Read the model definition and answer for the solid it produces. Units are mm, in the model's axes. Face numbers are marked on the shaded views. A direction names the side the tool comes from. Round coordinates to 2 decimals unless told otherwise and drop trailing zeros. Loops run counter-clockwise (first coordinate to the right, second up) from the corner with the lowest first, then second, coordinate; pieces in that order, holes last. Notation, with made-up numbers: M -31,-3.75 L 10,-3.75 A8 cw 10,1.25 Z; hole C 3,28 d3. An arc over 180 degrees is marked long. Answer as CSV lines item,"result".
```python
from build123d import *

# Parameters (mm, degrees)
CROQUIS1_R              = 4.05
SALIENTE_EXTRUIR1_DEPTH = 15
CORTAR_EXTRUIR1_REACH   = 10
CROQUIS2_R              = 2.5
REDONDEO1_R             = 0.5
REDONDEO2_R             = 0.1


with BuildPart() as part:
    # Croquis1 → Saliente-Extruir1 (new body, symmetric)
    with BuildSketch(Plane.XY):
        with BuildLine():
            Line((21, 0), (-21, 0))
            Line((-21, 0), (-21, 8))
            Line((-21, 8), (-12, 8))
            Line((-12, 8), (-12, 20))
            ThreePointArc((-12, 20), (0, 32), (12, 20))
            Line((12, 20), (12, 8))
            Line((12, 8), (21, 8))
            Line((21, 8), (21, 0))
        make_face()
        with Locations((0, 20)):
            Circle(CROQUIS1_R, mode=Mode.SUBTRACT)
    extrude(amount=SALIENTE_EXTRUIR1_DEPTH, both=True)

    # Croquis2 → Cortar-Extruir1 (cut, up to next)
    with BuildSketch(Plane(origin=(0, 8, 0), x_dir=(1, 0, 0), z_dir=(0, 1, 0)), mode=Mode.PRIVATE) as cortar_extruir1_sk1:
        with Locations((-17.5, 11.25)):
            Circle(CROQUIS2_R)
    cortar_extruir1_tool1 = extrude(cortar_extruir1_sk1.sketch, amount=-CORTAR_EXTRUIR1_REACH, mode=Mode.PRIVATE) & part.part
    add(cortar_extruir1_tool1.solids().sort_by_distance((-17.5, 8, -11.25))[0], mode=Mode.SUBTRACT)
    # Croquis2 → Cortar-Extruir1 (cut, up to next)
    with BuildSketch(Plane(origin=(0, 8, 0), x_dir=(1, 0, 0), z_dir=(0, 1, 0)), mode=Mode.PRIVATE) as cortar_extruir1_sk2:
        with Locations((17.5, 11.25)):
            Circle(CROQUIS2_R)
    cortar_extruir1_tool2 = extrude(cortar_extruir1_sk2.sketch, amount=-CORTAR_EXTRUIR1_REACH, mode=Mode.PRIVATE) & part.part
    add(cortar_extruir1_tool2.solids().sort_by_distance((17.5, 8, -11.25))[0], mode=Mode.SUBTRACT)
    # Croquis2 → Cortar-Extruir1 (cut, up to next)
    with BuildSketch(Plane(origin=(0, 8, 0), x_dir=(1, 0, 0), z_dir=(0, 1, 0)), mode=Mode.PRIVATE) as cortar_extruir1_sk3:
        with Locations((-17.5, -11.25)):
            Circle(CROQUIS2_R)
    cortar_extruir1_tool3 = extrude(cortar_extruir1_sk3.sketch, amount=-CORTAR_EXTRUIR1_REACH, mode=Mode.PRIVATE) & part.part
    add(cortar_extruir1_tool3.solids().sort_by_distance((-17.5, 8, 11.25))[0], mode=Mode.SUBTRACT)
    # Croquis2 → Cortar-Extruir1 (cut, up to next)
    with BuildSketch(Plane(origin=(0, 8, 0), x_dir=(1, 0, 0), z_dir=(0, 1, 0)), mode=Mode.PRIVATE) as cortar_extruir1_sk4:
        with Locations((17.5, -11.25)):
            Circle(CROQUIS2_R)
    cortar_extruir1_tool4 = extrude(cortar_extruir1_sk4.sketch, amount=-CORTAR_EXTRUIR1_REACH, mode=Mode.PRIVATE) & part.part
    add(cortar_extruir1_tool4.solids().sort_by_distance((17.5, 8, 11.25))[0], mode=Mode.SUBTRACT)

    # Redondeo1
    redondeo1_edges = [part.edges().sort_by_distance(p)[0] for p in [
        (12, 14, -15),
        (16.5, 8, 15),
        (21, 4, 15),
        (-21, 4, 15),
        (-16.5, 8, 15),
        (-12, 14, 15),
        (0, 32, 15),
        (12, 14, 15),
        (0, 32, -15),
        (12, 8, 0),
        (21, 8, 0),
        (-21, 8, 0),
        (-12, 8, 0),
        (-12, 14, -15),
        (-16.5, 8, -15),
        (-21, 4, -15),
        (21, 4, -15),
        (16.5, 8, -15),
    ]]
    fillet(redondeo1_edges, radius=REDONDEO1_R)

    # Redondeo2
    redondeo2_edges = [part.edges().sort_by_distance(p)[0] for p in [
        (-4.05, 20, 15),
        (-4.05, 20, -15),
    ]]
    fillet(redondeo2_edges, radius=REDONDEO2_R)


solid = part.part
```
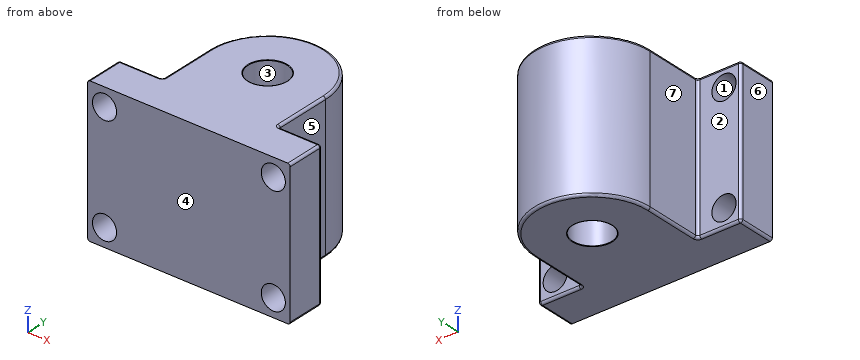
1) A tool of negligible diameter and unlimited length cuts with its end or side. For the marked faces 5, 6 and 7, from which of +Z, -Z, +X, -X, +Y, -Y can it reach the whole face along a straight path? Write none if from no direction.
Evaluation:
face 5,"+Z, -Z, +X, +Y"
face 6,"+Z, -Z, -X, +Y, -Y"
face 7,"+Z, -Z, -X, +Y"
2) Each of these flat-tipped pins is pushed along its axis until it touches: P1, Ø2, axis at x = 8, z = -0.5, coming from the +Y side; P2, Ø6.5, axis at x = -16, z = 7, coming from the +Y side; P3, Ø10, axis at x = 14.5, z = 10.5, coming from the +Y side. Where does it stop, or does it pass through?
Evaluation:
P1,"stops at y = 29.75"
P2,"stops at y = 8"
P3,"stops at y = 27.33"
3) Straight lines are drawn through the part: line 1 (X direction, y = 5, z = -11.5); line 2 (Z direction, x = 17.5, y = 6.25); line 3 (X direction, y = 11.5, z = -4.25). For each, find the intervals that lie inside material, in ascending order.
Evaluation:
line 1,"x = -21 to -19.99, -15.01 to 15.01, 19.99 to 21"
line 2,"z = -15 to -13.75, -8.75 to 8.75, 13.75 to 15"
line 3,"x = -12 to 12"
4) Find section C-C, the plane x = 17.5. Give the vertices of the cut face in (y, z), then the cut area to 3 significant figures.
Evaluation:
outline,"M 0,-15 L 7.5,-15 A0.5 ccw 8,-14.5 L 8,-13.75 L 0,-13.75 Z; M 0,-8.75 L 8,-8.75 L 8,8.75 L 0,8.75 Z; M 0,13.75 L 8,13.75 L 8,14.5 A0.5 ccw 7.5,15 L 0,15 Z"
area,"160 mm^2"
5) Find section A-A, the plane z = 11.25. Give the vertices of the cut face in (x, y), then the cut area to 3 significant figures.
Evaluation:
outline,"M -21,0 L -20,0 L -20,8 L -20.5,8 A0.5 ccw -21,7.5 Z; M -15,0 L 15,0 L 15,8 L 12.5,8 A0.5 cw 12,8.5 L 12,20 A12 ccw -12,20 L -12,8.5 A0.5 cw -12.5,8 L -15,8 Z; M 20,0 L 21,0 L 21,7.5 A0.5 ccw 20.5,8 L 20,8 Z; hole C 0,20 d8.1"
area,"719 mm^2"
6) Find section D-D, the plane z = 7.75. Give the vertices of the cut face in (x, y), then the cut area to 3 significant figures.
Evaluation:
outline,"M -21,0 L 21,0 L 21,7.5 A0.5 ccw 20.5,8 L 12.5,8 A0.5 cw 12,8.5 L 12,20 A12 ccw -12,20 L -12,8.5 A0.5 cw -12.5,8 L -20.5,8 A0.5 ccw -21,7.5 Z; hole C 0,20 d8.1"
area,"799 mm^2"
7) Find section B-B, the plane x = 0. Give the vertices of the cut face in (y, z).
Evaluation:
outline,"M 0,-15 L 15.85,-15 A0.1 ccw 15.95,-14.9 L 15.95,14.9 A0.1 ccw 15.85,15 L 0,15 Z; M 24.05,-14.9 A0.1 ccw 24.15,-15 L 31.5,-15 A0.5 ccw 32,-14.5 L 32,14.5 A0.5 ccw 31.5,15 L 24.15,15 A0.1 ccw 24.05,14.9 Z"
8) Determine the mould class of the marked faces 1, 2, 3 and 4 for opening direction Y: released by +Y, released by -Y, zero draft, split by the parting line, or undercut.
Evaluation:
face 1,"zero draft"
face 2,"released by +Y"
face 3,"undercut"
face 4,"released by -Y"
